```python
from build123d import *

# Parameters (mm, degrees)
EXTRUDE_1_DEPTH     = 6
FILLET_1_R          = 3
FILLET_2_R          = 1
SKETCH_2_R          = 1.25
CUT_EXTRUDE_1_DEPTH = 20.899748742
FILLET_3_R          = 1


# Some blends are built 0.0001 mm under size
with BuildPart() as part:
    # Эскиз1 → Бобышка-Вытянуть1 (new body)
    with BuildSketch(Plane(origin=(0, 0, 0), x_dir=(1, 0, 0), z_dir=(0, 1, 0))):
        Polygon((0, 0), (0, 5), (4, 5), (4, 12), (0, 12), (0, 18), (6, 18), (6, 2), (1, 2), (1, 0), align=None)
    extrude(amount=EXTRUDE_1_DEPTH)

    # Скругление1
    fillet_1_edges = [part.edges().sort_by_distance(p)[0] for p in [
        (3, 0, -18),
        (3, 6, -18),
    ]]
    fillet(fillet_1_edges, radius=FILLET_1_R - 0.0001)  # a hair under: the kernel refuses the full size

    # Скругление2
    fillet_2_edges = [part.edges().sort_by_distance(p)[0] for p in [
        (3.5, 6, -2),
        (4, 0, -8.5),
        (2, 0, -12),
        (6, 0, -8.50005),
        (3.5, 0, -2),
        (6, 6, -8.50005),
        (0, 3, -5),
        (4, 3, -5),
        (4, 3, -12),
        (6, 3, -2),
        (2, 6, -12),
        (4, 6, -8.5),
        (2, 6, -5),
        (6, 5.121349633, -17.121349633),
        (6, 0.878650367, -17.121349633),
        (2, 0, -5),
    ]]
    fillet(fillet_2_edges, radius=FILLET_2_R - 0.0001)  # a hair under: the kernel refuses the full size

    # Эскиз2 → Вырез-Вытянуть1 (cut, through all)
    with BuildSketch(Plane.ZY):
        with Locations((-15, 3)):
            Circle(SKETCH_2_R)
    extrude(amount=-CUT_EXTRUDE_1_DEPTH, mode=Mode.SUBTRACT)

    # Скругление3
    # the kernel refuses this fillet: 1 mm, written as the material it takes off along each edge
    with BuildSketch(Plane(origin=(6, 3, -15), x_dir=(0, 0, 1), z_dir=(0, -1, 0))) as fillet_3_piece_1:
        with BuildLine():
            CenterArc((1.25 + FILLET_3_R, FILLET_3_R), FILLET_3_R, 180, 90)
            Line((1.25 + FILLET_3_R, 0), (1.25, 0))
            Line((1.25, 0), (1.25, FILLET_3_R))
        make_face()
    revolve(axis=Axis((6, 3, -15), (-1, 0, 0)), mode=Mode.SUBTRACT)


solid = part.part
```
Work out the finished part from the listing and answer in its coordinate system (mm). A direction names the side the tool comes from. Give positions to 0.01 mm unless a question says otherwise; leave off trailing zeros. Loops run counter-clockwise (first coordinate to the right, second up) from the corner with the lowest first, then second, coordinate; pieces in that order, holes last. Notation, with made-up numbers: (7.25, 37) -> (14.25, 37) arc R29 cw to (14.25, 61) -> close; hole circle Ø2 at (-1, 70.5). An arc over 180 degrees is marked (long way). Write item = value, one per line. Start each with the question number.
(1) Find the intervals of material crossed by probe 1 along Y at (x, z) = (1.15, -15); probe 2 along Z at (x, y) = (1.5, 3.25); probe 3 along X at (y, z) = (3.5, -10.25), in increasing order. Write a range as from..to.
(2) Find section C-C on z = -2.25. Give the vertices of the cut face in (x, y).
(3) The mould has two halves that part along Y. Classify faces 4 (the flat face through (4, 6, -13)), 5 (the cylindrical face through (2.46, 3.05, -16.25)), 6 (the cylindrical face through (1.521, 0.285, -4.699)): +Y half, -Y half, draft (parallel to the pull), parting line (faces both ways), or undercut.
(4) Find section A-A on x = 1.25. Give the number of separate pieces and of enclosed holes in the cut face, and give its area (3 significant figures).
(5) Which of the six approach directions +Z, -Z, +X, -X, +Y, -Y give full straight-line access (tool end or side, diameter ignored) to faces 1 (the flat face through (3, 3, -2)), 2 (the cylindrical face through (4.301, 5.715, -8.535)), 3 (the cylindrical face through (1.479, 0.285, -12.301))?
(6) Given pin 1 Ø1.2 at (y, z) = (2, -8.5) entering from -X; pin 2 Ø2 at (x, y) = (4.5, 1.5) entering from +Z; pin 3 Ø0.6 at (x, y) = (2, 3.5) entering from -Z, each flat-ended and moving along its own axis, determine where each tip first touches the part or whether it passes through.
From the geometry:
q1.probe_1 = 0..1.75, 4.25..6
q1.probe_2 = -17.99..-16.22, -13.78..-12, -5..-2
q1.probe_3 = 4..6
q2.outline = (0, 0) -> (1, 0) -> (1, 0.34) -> (5, 0.34) arc R0.66 ccw to (5.66, 1) -> (5.66, 5) arc R0.66 ccw to (5, 5.66) -> (1, 5.66) -> (1, 6) -> (0, 6) -> close
q3.face_4 = +Y half
q3.face_5 = undercut
q3.face_6 = -Y half
q4.separate_pieces = 2
q4.enclosed_holes = 1
q4.area = 43.9 mm^2
q5.face_1 = +Z, +X, +Y, -Y
q5.face_2 = -X, +Y
q5.face_3 = -X, -Y
q6.pin_1 = 4
q6.pin_2 = -2
q6.pin_3 = -17.99
